from build123d import *

# Parameters (mm, degrees)
SKETCH1_W                    = 30
SKETCH1_H                    = 394
BASE_FLANGE1_DEPTH           = 2
EDGE_FLANGE1_STRIP_W         = 13
EDGE_FLANGE1_STRIP_H         = 2
EDGE_FLANGE1_STRIP_CUT_DEPTH = 394
EDGE_FLANGE1_DEPTH           = 394


# Sheet-metal steps are written as plain solids
with BuildPart() as part:
    # Sketch1 → Base-Flange1 (new body)
    with BuildSketch(Plane(origin=(0, 0, 0), x_dir=(0, 0, -1), z_dir=(1, 0, 0))):
        Rectangle(SKETCH1_W, SKETCH1_H)
    extrude(amount=-BASE_FLANGE1_DEPTH)

    # Edge-Flange1 strip (across the edge) → Edge-Flange1 strip cut (cut)
    with BuildSketch(Plane(origin=(0, -197, -15), x_dir=(0, 0, 1), z_dir=(0, 1, 0))):
        with Locations((-2, -1)):
            Rectangle(EDGE_FLANGE1_STRIP_W, EDGE_FLANGE1_STRIP_H)
    extrude(amount=EDGE_FLANGE1_STRIP_CUT_DEPTH, mode=Mode.SUBTRACT)

    # Edge-Flange1 section (across the edge) → Edge-Flange1 (add)
    with BuildSketch(Plane(origin=(0, -197, -15), x_dir=(0, 0, 1), z_dir=(0, 1, 0))):
        with BuildLine():
            Line((0, 2.5), (0, 28))
            Line((0, 28), (2, 28))
            Line((2, 28), (2, 2.5))
            ThreePointArc((2, 2.5), (2.732233047, 0.732233047), (4.5, 0))
            Line((4.5, 0), (4.5, -2))
            ThreePointArc((4.5, -2), (1.318019485, -0.681980515), (0, 2.5))
        make_face()
    extrude(amount=EDGE_FLANGE1_DEPTH)


solid = part.part
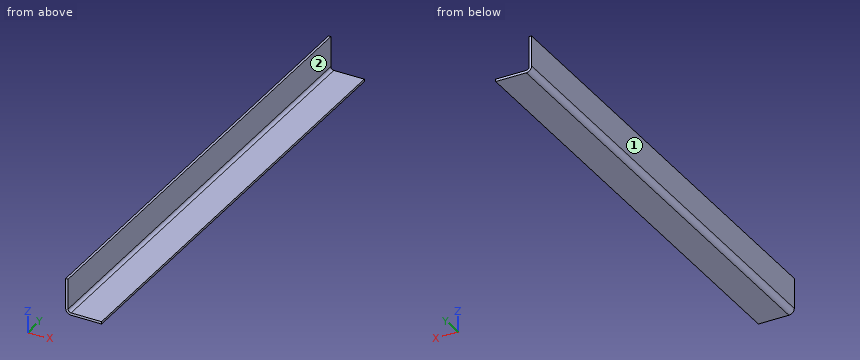
The listing builds one solid part. Answer for the finished solid, in the listing's coordinates (mm). Face numbers are marked on the shaded views. A direction names the side the tool comes from. Round coordinates to 2 decimals unless told otherwise and drop trailing zeros. Order: outer loops, then holes, each group sorted by start corner. A loop starts at its lowest first (then second) coordinate and runs counter-clockwise, first axis right, second up. Notation, with made-up numbers: (23.5, 66.5) -> (27.5, 66.5) arc R29 cw to (27.5, 86.5) -> close; hole circle Ø10 at (-37.75, -13.75). An arc over 180 degrees is marked (long way). One line per item, written item: value.
Item 1: Find section A-A, the plane y = -36. Give the vertices of the cut face in (x, z).
Taken from the geometry:
outline: (-2, -10.5) arc R4.5 ccw to (2.5, -15) -> (28, -15) -> (28, -13) -> (2.5, -13) arc R2.5 cw to (0, -10.5) -> (0, 15) -> (-2, 15) -> close
Item 2: Find section B-B, the plane x = 23.25. Give the vertices of the cut face in (y, z), then the cut area to 3 significant figures.
Taken from the geometry:
outline: (-197, -15) -> (197, -15) -> (197, -13) -> (-197, -13) -> close
area: 788 mm2
Item 3: For the marked faces 1 and 2, determine the directions among +Z, -Z, +X, -X, +Y, -Y from which every point of the face is accessible in a straight line to the end or side of a thin tool.
Taken from the geometry:
face 1: +Z, -Z, -X, +Y, -Y
face 2: +Z, +X, +Y, -Y
Item 4: Straight lines are drawn through the part: L1, parallel to X at y = 130, z = 10.75; L2, parallel to Z at x = 22.5, y = 142; L3, parallel to X at y = 159.5, z = -12.25. For each, find the intervals that lie inside material, in ascending order.
Taken from the geometry:
L1: x = -2 to 0
L2: z = -15 to -13
L3: x = -1.65 to 0.71
Item 5: Find section C-C, the plane z = 10. Give the vertices of the cut face in (x, y).
Taken from the geometry:
outline: (-2, -197) -> (0, -197) -> (0, 197) -> (-2, 197) -> close
Item 6: Given P1, Ø1.5, axis at x = 10, y = -138, coming from the +Z side, flat-ended and moving along its own axis, determine where the tip first touches the part or whether it passes through.
Taken from the geometry:
P1: stops at z = -13
